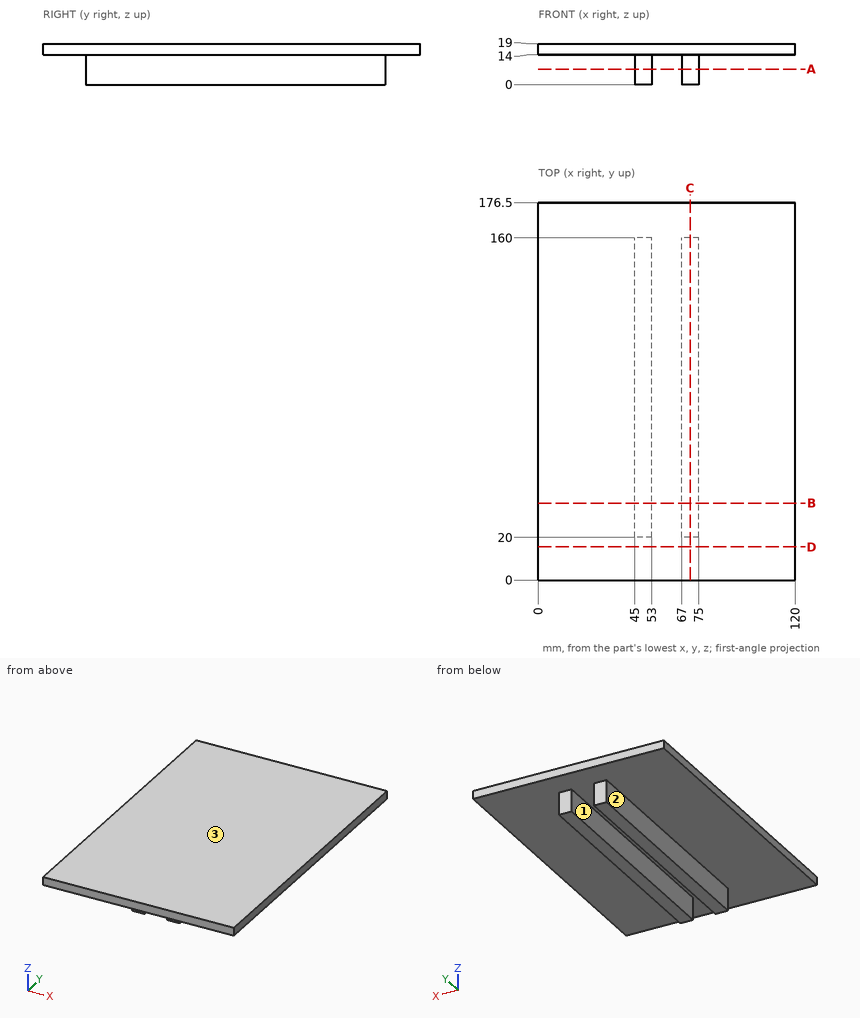
The drawing under review shows one solid part. Ordinate dimensions are in mm from its lowest x, y, z. Give positions to 0.01 mm unless a question says otherwise; leave off trailing zeros. Write each loop counter-clockwise with the first axis right and the second up, starting at its lowest first coordinate (ties: lowest second). Pieces come first, ordered by that corner, then holes. Notation, with made-up numbers: (31.5, 64.25) - (85.5, 64.25) arc R26 cw to (85.5, 78.25) - close; hole circle Ø5 at (85.5, -32). An arc over 180 degrees is marked (long way). Answer in a Markdown table with one row per item. Add a question column.
1. We need section D-D on y = 15.5. Write out the cut boundary in (x, z).
2. We need section C-C on x = 71. Write out the cut boundary in (y, z).
3. Insertion check: P1, Ø6, axis at x = 71, z = 8.5, coming from the +Y side; P2, Ø10, axis at y = 154.5, z = 7, coming from the +X side; P3, Ø6.5, axis at x = 51, z = 7, coming from the -Y side. Each pin has a flat end and moves straight along its axis. Give the tip position at first contact, or say it passes through.
4. Wall thickness on line 1 along X through (y, z) = (56, 9.5); line 2 along Z through (x, y) = (14.5, 99); line 3 along Y through (x, z) = (69, 7.5): over which ranges is each line inside the solid? List them lowest first. Write a range as [from, to].
5. We need section B-B on y = 36. Write out the cut boundary in (x, z), then the cut area to 3 significant figures.
6. Draft analysis for pull direction X (two halves, no side actions). For the marked faces 1, 2 and 3, state which applies: +X half, -X half, draft (parallel to the pull), parting line (faces both ways), or undercut.
7. We need section A-A on z = 7.25. Write out the cut boundary in (x, y), then the cut area to 3 significant figures.
Ans:
| question | item | result |
|---|---|---|
| 1 | outline | (0, 14) - (120, 14) - (120, 19) - (0, 19) - close |
| 2 | outline | (0, 14) - (20, 14) - (20, 0) - (160, 0) - (160, 14) - (176.5, 14) - (176.5, 19) - (0, 19) - close |
| 3 | P1 | stops at y = 160 |
| 3 | P2 | stops at x = 75 |
| 3 | P3 | stops at y = 20 |
| 4 | line 1 | x = [45, 53], [67, 75] |
| 4 | line 2 | z = [14, 19] |
| 4 | line 3 | y = [20, 160] |
| 5 | outline | (0, 14) - (45, 14) - (45, 0) - (53, 0) - (53, 14) - (67, 14) - (67, 0) - (75, 0) - (75, 14) - (120, 14) - (120, 19) - (0, 19) - close |
| 5 | area | 824 mm^2 |
| 6 | face 1 | undercut |
| 6 | face 2 | -X half |
| 6 | face 3 | draft |
| 7 | outline | (45, 20) - (53, 20) - (53, 160) - (45, 160) - close; (67, 20) - (75, 20) - (75, 160) - (67, 160) - close |
| 7 | area | 2,240 mm^2 |
